```python
from build123d import *

# Parameters (mm, degrees)
F1_DEPTH = 25.4
F2_R     = 8.89
F3_DEPTH = 97.9802
F5_DEPTH = 98.298
F6_W     = 76.2
F6_H     = 127
F7_DEPTH = 12.7
F9_DEPTH = 25.4


with BuildPart() as f1:
    # F0 (on Front) → F1 (new body)
    with BuildSketch(Plane.XZ):
        with BuildLine():
            ThreePointArc((-25.4, 72.847709), (0, 98.247709), (25.4, 72.847709))
            Line((25.4, 72.847709), (25.4, -3.352291))
            Line((25.4, -3.352291), (38.1, -3.352291))
            Line((38.1, -3.352291), (38.1, 72.847709))
            ThreePointArc((38.1, 72.847709), (31.10852, 94.844754), (12.7, 108.768733))
            Line((12.7, 108.768733), (12.7, 123.647709))
            Line((12.7, 123.647709), (0, 123.647709))
            Line((0, 123.647709), (-12.7, 123.647709))
            Line((-12.7, 123.647709), (-12.7, 108.768733))
            ThreePointArc((-12.7, 108.768733), (-31.10852, 94.844754), (-38.1, 72.847709))
            Line((-38.1, 72.847709), (-38.1, -3.352291))
            Line((-38.1, -3.352291), (-25.4, -3.352291))
            Line((-25.4, -3.352291), (-25.4, 72.847709))
        make_face()
    extrude(amount=F1_DEPTH)

    # F2 (on face) → F3 (cut)
    with BuildSketch(Plane.XY.offset(123.647709)):
        with Locations((0, -12.7)):
            Circle(F2_R)
    extrude(amount=-F3_DEPTH, mode=Mode.SUBTRACT)

    # F4 (on Top) → F5 (cut)
    with BuildSketch(Plane.XY):
        with BuildLine():
            Line((8.89, -21.59), (8.89, -12.7))
            ThreePointArc((8.89, -12.7), (6.286179, -18.986179), (0, -21.59))
            Line((0, -21.59), (8.89, -21.59))
        make_face()
        with BuildLine():
            ThreePointArc((0, -3.81), (6.286179, -6.413821), (8.89, -12.7))
            Line((8.89, -12.7), (8.89, -3.81))
            Line((8.89, -3.81), (0, -3.81))
        make_face()
        with BuildLine():
            ThreePointArc((-8.89, -12.7), (-6.286179, -6.413821), (0, -3.81))
            Line((0, -3.81), (-8.89, -3.81))
            Line((-8.89, -3.81), (-8.89, -12.7))
        make_face()
        with BuildLine():
            Line((-8.89, -21.59), (0, -21.59))
            ThreePointArc((0, -21.59), (-6.286179, -18.986179), (-8.89, -12.7))
            Line((-8.89, -12.7), (-8.89, -21.59))
        make_face()
    extrude(amount=F5_DEPTH, mode=Mode.SUBTRACT)

    # F6 (on face) → F7 (join)
    with BuildSketch(Plane(origin=(0, 0, -3.352291), x_dir=(1, 0, 0), z_dir=(0, 0, -1))):
        with Locations((0, -38.1)):
            Rectangle(F6_W, F6_H)
    extrude(amount=F7_DEPTH)

    # F8 (on face) → F9 (join)
    with BuildSketch(Plane.XZ.offset(25.4)):
        Polygon((0, -16.052291), (38.1, -16.052291), (38.1, -3.352291), (0, -3.352291), (-38.1, -3.352291), (-38.1, -16.052291), align=None)
    extrude(amount=F9_DEPTH)


solid = f1.part
```
Geometry: final body of the model. Coordinates: model frame, mm. A direction names the side the tool comes from. Coordinates: 2 decimals unless noted, no trailing zeros. Order: outer loops, then holes, each group sorted by start corner. A loop starts at its lowest first (then second) coordinate and runs counter-clockwise, first axis right, second up. Notation, with made-up numbers: (78.25, 71.25) - (112.25, 71.25) arc R7 ccw to (112.25, 83.25) - close; hole circle Ø9 at (-40, 58.5). An arc over 180 degrees is marked (long way). Write each question's results on one line, items separated by ' | '.
(1) Section query A-A, the plane z = 58.5. Return the cut outline in (x, y).
Values found:
outline: (-38.1, -25.4) - (-25.4, -25.4) - (-25.4, 0) - (-38.1, 0) - close; (25.4, -25.4) - (38.1, -25.4) - (38.1, 0) - (25.4, 0) - close
(2) Section query B-B, the plane x = -22. Return the cut outline in (y, z).
Values found:
outline: (-50.8, -16.05) - (101.6, -16.05) - (101.6, -3.35) - (-50.8, -3.35) - close; (-25.4, 85.54) - (0, 85.54) - (0, 103.95) - (-25.4, 103.95) - close
(3) Section query D-D, the plane x = 28. Return the cut outline in (y, z).
Values found:
outline: (-50.8, -16.05) - (101.6, -16.05) - (101.6, -3.35) - (0, -3.35) - (0, 98.69) - (-25.4, 98.69) - (-25.4, -3.35) - (-50.8, -3.35) - close
(4) Set-up query: faces 1 (the face through (-25.4, -13, 34)), 2 (the face through (7, -6, 98.298)), 3 (the face through (-26, -25.4, 70)), 4 (the face through (-12.7, -13, 116)). Return all of +Z, -Z, +X, -X, +Y, -Y with unobstructed straight access to the full face (end or side cutting, diameter ignored); none if empty.
Values found:
face 1: +Y, -Y | face 2: none | face 3: +Z, +X, -X, -Y | face 4: +Z, -X, +Y, -Y
(5) Line query: line 1 (Y direction, x = 0, z = 108); line 2 (X direction, y = -11.5, z = 66.5); line 3 (Z direction, x = -26, y = 13.5). Output: solid intervals per line, ascending. Write a range as [from, to].
Values found:
line 1: y = [-25.4, -21.59], [-3.81, 0] | line 2: x = [-38.1, -25.4], [25.4, 38.1] | line 3: z = [-16.05, -3.35]
(6) Section query C-C, the plane y = 60.5. Return the cut outline in (x, z).
Values found:
outline: (-38.1, -16.05) - (38.1, -16.05) - (38.1, -3.35) - (-38.1, -3.35) - close
(7) First-contact query: pin 1 Ø12 at (y, z) = (-8, 115.5) entering from +X; pin 2 Ø2 at (x, y) = (17, 14) entering from +Z; pin 3 Ø16.5 at (y, z) = (-9, 118) entering from -X; pin 4 Ø6 at (x, y) = (13, 1.5) entering from +Z. Flat tips, straight axial feed; report the tip coordinate or a pass-through.
Values found:
pin 1: stops at x = 12.7 | pin 2: stops at z = -3.35 | pin 3: stops at x = -12.7 | pin 4: stops at z = 123.65
(8) Mould query, pull axis X, two halves, no side actions, for faces 5 (the face through (12.7, -13, 116)), 6 (the face through (3, -4, 123.648)), 7 (the face through (-7, -6, 98.298)). Classes: +X half, -X half, draft (parallel to the pull), parting line (faces both ways), or undercut.
Values found:
face 5: +X half | face 6: draft | face 7: undercut
